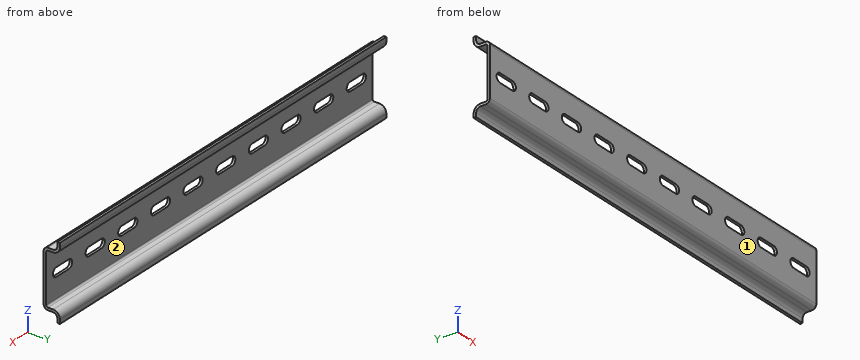
```python
from build123d import *

# Parameters (mm, degrees)
EXTRUDE_THIN1_DEPTH = 101.6
CUT_EXTRUDE1_DEPTH  = 1.2
LPATTERN1_COUNT     = 10
LPATTERN1_PITCH     = 20.32


with BuildPart() as part:
    # Sketch1 → Extrude-Thin1 (new body, symmetric)
    with BuildSketch(Plane(origin=(0, 0, 0), x_dir=(0, 0, -1), z_dir=(1, 0, 0))):
        with BuildLine():
            Line((-17.5, 6.5), (-15.5, 6.5))
            ThreePointArc((-15.5, 6.5), (-14.085786438, 5.914213562), (-13.5, 4.5))
            Line((-13.5, 4.5), (-13.5, 2))
            ThreePointArc((-13.5, 2), (-12.914213562, 0.585786438), (-11.5, 0))
            Line((-11.5, 0), (11.5, 0))
            ThreePointArc((11.5, 0), (12.914213562, 0.585786438), (13.5, 2))
            Line((13.5, 2), (13.5, 4.5))
            ThreePointArc((13.5, 4.5), (14.085786438, 5.914213562), (15.5, 6.5))
            Line((15.5, 6.5), (17.5, 6.5))
            Line((17.5, 6.5), (17.5, 7.7))
            Line((17.5, 7.7), (15.5, 7.7))
            ThreePointArc((15.5, 7.7), (13.2372583, 6.7627417), (12.3, 4.5))
            Line((12.3, 4.5), (12.3, 2))
            ThreePointArc((12.3, 2), (12.065685425, 1.434314575), (11.5, 1.2))
            Line((11.5, 1.2), (-11.5, 1.2))
            ThreePointArc((-11.5, 1.2), (-12.065685425, 1.434314575), (-12.3, 2))
            Line((-12.3, 2), (-12.3, 4.5))
            ThreePointArc((-12.3, 4.5), (-13.2372583, 6.7627417), (-15.5, 7.7))
            Line((-15.5, 7.7), (-17.5, 7.7))
            Line((-17.5, 7.7), (-17.5, 6.5))
        make_face()
    extrude(amount=EXTRUDE_THIN1_DEPTH, both=True)

    # Sketch2 → Cut-Extrude1 (cut)
    with BuildSketch(Plane.XZ):
        with BuildLine():
            Line((87.54, 2.1), (95.34, 2.1))
            ThreePointArc((95.34, 2.1), (97.44, 0), (95.34, -2.1))
            Line((95.34, -2.1), (87.54, -2.1))
            ThreePointArc((87.54, -2.1), (85.44, 0), (87.54, 2.1))
        make_face()
    cut_extrude1 = extrude(amount=-CUT_EXTRUDE1_DEPTH, mode=Mode.SUBTRACT)

    # LPattern1: Cut-Extrude1 ×10
    with Locations(*[(-i * LPATTERN1_PITCH, 0, 0) for i in range(1, LPATTERN1_COUNT)]):
        add(cut_extrude1, mode=Mode.SUBTRACT)


solid = part.part
```
Check sheet for the modelled part. Datum: model origin and axes. Units: mm. Face numbers are marked on the shaded views. Coordinates: 2 decimals unless noted, no trailing zeros. Order: outer loops, then holes, each group sorted by start corner. A loop starts at its lowest first (then second) coordinate and runs counter-clockwise, first axis right, second up. Notation, with made-up numbers: (7, 0) -> (63, 0) arc R19 cw to (63, 11) -> close; hole circle Ø10 at (83, 19). An arc over 180 degrees is marked (long way). Write each question's results on one line, items separated by ' | '. Start each with the question number.
1) Draft check along Z on the marked faces 1 and 2. Enter one of: pulls with the +Z half, pulls with the -Z half, needs draft (parallel to the pull), parting line crosses it, or undercut.
2) Material ranges on line 1 along Z through (x, y) = (54, 4); line 2 along Z through (x, y) = (28.5, 7); line 3 along Y through (x, z) = (16, 2), recorded low to high.
3) Section check B-B (x = 39). Enter the section's corners in (y, z), and give its area (3 significant figures).
4) Section check C-C (z = -4). Enter the section's corners in (x, y).
5) Depth check by flat-ended pin: pin 1 (1.2 mm diameter, centred on x = 29.5, y = 3, fed in from +Z); pin 2 (2 mm diameter, centred on x = -2.5, y = 4.5, fed in from +Z); pin 3 (1.2 mm diameter, centred on x = 11.5, y = 3, fed in from -Z); pin 4 (3 mm diameter, centred on y = 3.5, z = -0.5, fed in from -X). Enter the tip coordinate at first touch or a pass-through.
6) Section check A-A (x = -69.5). Enter the section's corners in (y, z).
Checked values:
1) face 1: needs draft | face 2: undercut
2) line 1: -13.5 to -12.3, 12.3 to 13.5 | line 2: -17.5 to -13.5, 13.5 to 17.5 | line 3: 0 to 1.2
3) outline: (0, -11.5) arc R2 ccw to (2, -13.5) -> (4.5, -13.5) arc R2 cw to (6.5, -15.5) -> (6.5, -17.5) -> (7.7, -17.5) -> (7.7, -15.5) arc R3.2 ccw to (4.5, -12.3) -> (2, -12.3) arc R0.8 cw to (1.2, -11.5) -> (1.2, 11.5) arc R0.8 cw to (2, 12.3) -> (4.5, 12.3) arc R3.2 ccw to (7.7, 15.5) -> (7.7, 17.5) -> (6.5, 17.5) -> (6.5, 15.5) arc R2 cw to (4.5, 13.5) -> (2, 13.5) arc R2 ccw to (0, 11.5) -> close | area: 53.5 mm²
4) outline: (-101.6, 0) -> (101.6, 0) -> (101.6, 1.2) -> (-101.6, 1.2) -> close
5) pin 1: z = 13.5 | pin 2: z = 13.77 | pin 3: z = -13.5 | pin 4: through
6) outline: (0, -11.5) arc R2 ccw to (2, -13.5) -> (4.5, -13.5) arc R2 cw to (6.5, -15.5) -> (6.5, -17.5) -> (7.7, -17.5) -> (7.7, -15.5) arc R3.2 ccw to (4.5, -12.3) -> (2, -12.3) arc R0.8 cw to (1.2, -11.5) -> (1.2, -2.1) -> (0, -2.1) -> close; (0, 2.1) -> (1.2, 2.1) -> (1.2, 11.5) arc R0.8 cw to (2, 12.3) -> (4.5, 12.3) arc R3.2 ccw to (7.7, 15.5) -> (7.7, 17.5) -> (6.5, 17.5) -> (6.5, 15.5) arc R2 cw to (4.5, 13.5) -> (2, 13.5) arc R2 ccw to (0, 11.5) -> close
